Check sheet for the modelled part. Datum: model origin and axes. Units: mm. A direction names the side the tool comes from. Coordinates: 2 decimals unless noted, no trailing zeros. Write each loop counter-clockwise with the first axis right and the second up, starting at its lowest first coordinate (ties: lowest second). Pieces come first, ordered by that corner, then holes. Notation, with made-up numbers: M -28.75,22 L 5.25,22 A17 ccw 5.25,43 Z; hole C 65,40 d11. An arc over 180 degrees is marked long. Answer as CSV lines item,"result". Start each with the question number.
Q1. Thickness scan on line 1 along X through (y, z) = (-15, 2.7); line 2 along Y through (x, z) = (-3.5, 3.4). Record the ranges inside material, lowest first. Write a range as from..to.
Q2. Access from +Z, -Z, +X, -X, +Y, -Y to the whole of each face (thin tool, end or side, straight path). Record for faces 5 (the flat face through (-25, 0, 2)), 6 (the conical face through (-65.979, 63.141, 3.125)).
Q3. Sectioned sample at C-C, the plane z = 3.9. Record the cut outline in (x, y), then the cut area to 3 significant figures.
Q4. Sectioned sample at A-A, the plane y = -21.5. Record the cut outline in (x, z).
Q5. Mould release check, pull along Y, two halves, no side actions. Record for faces 1 (the flat face through (75, -1, 2)), 2 (the flat face through (0, -25, 2)), 3 (the flat face through (-1, 75, 2)), 4 (the conical face through (-65.979, -65.119, 3.125)): pulls with the +Y half, pulls with the -Y half, needs draft (parallel to the pull), parting line crosses it, or undercut.
Q6. Depth check by flat-ended pin: pin 1 Ø5 at (x, y) = (-64.69, 64.13) entering from +Z; pin 2 Ø3.5 at (x, y) = (64.69, 64.13) entering from +Z; pin 3 Ø4 at (x, y) = (-64.69, -64.13) entering from +Z. Enter the tip coordinate at first touch or a pass-through.
from build123d import *

# Parameters (mm, degrees)
F0_W     = 150
F0_H     = 150
F0_R     = 1.5
F1_DEPTH = 5
F2_SIZE  = 2


with BuildPart() as f1:
    # F0 (on Top) → F1 (new body)
    with BuildSketch(Plane.XY):
        Rectangle(F0_W, F0_H)
        with Locations((-64.68948, -64.129733)):
            Circle(F0_R, mode=Mode.SUBTRACT)
        with Locations((64.68948, -64.129733)):
            Circle(F0_R, mode=Mode.SUBTRACT)
        with Locations((-64.68948, 64.129733)):
            Circle(F0_R, mode=Mode.SUBTRACT)
        Polygon((-25, -25), (-25, 25), (-13, 25), (-13, 37), (13, 37), (13, 25), (25, 25), (25, -25), align=None, mode=Mode.SUBTRACT)
        with Locations((64.68948, 64.129733)):
            Circle(F0_R, mode=Mode.SUBTRACT)
    extrude(amount=F1_DEPTH)

    # F2
    f2_edges = [f1.edges().sort_by_distance(p)[0] for p in [
        (-66.18948, 64.129733, 5),
        (-66.18948, -64.129733, 5),
        (63.18948, -64.129733, 5),
        (63.18948, 64.129733, 5),
    ]]
    chamfer(f2_edges, length=F2_SIZE)


solid = f1.part
Output:
1,line 1,"x = -75..-25, 25..75"
1,line 2,"y = -75..-25, 37..75"
2,face 5,"+Z, -Z"
2,face 6,"+Z"
3,outline,"M -75,-75 L 75,-75 L 75,75 L -75,75 Z; hole C -64.69,-64.13 d4.8; hole C -64.69,64.13 d4.8; hole M -25,-25 L 25,-25 L 25,25 L 13,25 L 13,37 L -13,37 L -13,25 L -25,25 Z; hole C 64.69,-64.13 d4.8; hole C 64.69,64.13 d4.8"
3,area,"19,600 mm^2"
4,outline,"M -75,0 L -25,0 L -25,5 L -75,5 Z; M 25,0 L 75,0 L 75,5 L 25,5 Z"
5,face 1,"needs draft"
5,face 2,"undercut"
5,face 3,"pulls with the +Y half"
5,face 4,"undercut"
6,pin 1,"stops at z = 4"
6,pin 2,"stops at z = 3.25"
6,pin 3,"stops at z = 3.5"
